The model under review builds one solid part; all positions refer to its coordinate system, in mm. A direction names the side the tool comes from. Give positions to 0.01 mm unless a question says otherwise; leave off trailing zeros. Loops run counter-clockwise (first coordinate to the right, second up) from the corner with the lowest first, then second, coordinate; pieces in that order, holes last. Notation, with made-up numbers: M 53,26 L 107,26 A16 ccw 107,47 Z; hole C 53,75.5 d8. An arc over 180 degrees is marked long. One line per item, written item: value. Start each with the question number.
Q1. Mouldability with a two-part tool opening along X and no side actions: class faces 3 (the face through (-30.2, 11.3, 0)), 4 (the face through (20.935, 16, -103)), 5 (the face through (-33.04, 14, -75)) as released by +X, released by -X, zero draft, split by the parting line, or undercut.
Q2. We need section C-C on x = -28. Write out the cut boundary in (y, z) (3 decimals).
Q3. For pin 1 (1 mm diameter, centred on x = -22.5, z = -66.5, fed in from +Y) (3 decimals); pin 2 (2 mm diameter, centred on y = 3.5, z = -43.5, fed in from +X); pin 3 (7.5 mm diameter, centred on y = 18.5, z = -52.5, fed in from +X), all flat-tipped, find the tip position at first contact; note any pin that passes through.
Q4. We need section B-B on z = -93.5. Write out the cut boundary in (x, y) (3 decimals), plus the area to 3 significant figures.
Q5. We need section D-D on z = -39.5. Write out the cut boundary in (x, y) (3 decimals), plus the area to 3 significant figures.
Q6. We need section A-A on y = 23. Write out the cut boundary in (x, z), plus the area to 3 significant figures.
Q7. For faces 1 (the face through (-5, 3.175, -92)), 2 (the face through (23, 28.575, -103)), list the 3-axis set-ups (+Z, -Z, +X, -X, +Y, -Y) from which the entire face can be reached by the end or side of a thin tool; tool diameter is ignored.
Q8. To check wall thickness, follow line 1 along X through (y, z) = (10, -85); line 2 along Y through (x, z) = (4, -50) (3 decimals); line 3 along X through (y, z) = (23.5, -7). State the ranges of each line that lie inside material, in increasing order. Write a range as from..to.
Autodesk Inventor part; units mm, degrees
ref_plane "YZ Plane" through (0, 0, 0) normal (1, 0, 0) x (0, 1, 0)
ref_plane "XZ Plane" through (0, 0, 0) normal (0, 1, 0) x (-1, 0, 0)
ref_plane "XY Plane" through (0, 0, 0) normal (0, 0, 1) x (1, 0, 0)
sketch "Sketch1" plane through (0, 0, 0) normal (0, 0, 1) x (1, 0, 0)
  line L0 (24.1101, 28.575) -> (24.1101, 0)
  line L1 (24.1101, 0) -> (-33.0399, 0)
  line L2 (-33.0399, 0) -> (-33.0399, 28.575)
  line L3 (-29.8649, 28.575) -> (-29.8649, 3.175)
  line L4 (-29.8649, 3.175) -> (20.9351, 3.175)
  line L5 (20.9351, 3.175) -> (20.9351, 28.575)
  line L6 (-33.0399, 28.575) -> (-29.8649, 28.575)
  line L7 (24.1101, 28.575) -> (20.9351, 28.575)
  point P0 (0, 0)
  dimension "d0" = 57.15
  dimension "d1" = 28.575
  dimension "d2" = 3.175
  dimension "d18" = 28.575
extrude "Extrusion1" add sketch "Sketch1" against normal blind 152.4
sketch "Sketch5" plane through (-33.0399, 0, 0) normal (0, -1, 0) x (1, 0, 0)
  line L0 (0, 0) -> (57.15, 0)
  line L1 (57.15, 0) -> (57.15, -152.4)
  line L2 (57.15, -152.4) -> (57.15, -59.69)
  line L3 (57.15, 0) -> (57.15, -152.4)
  line L4 (57.15, -59.69) -> (10.5151, 0)
  line L5 (10.5151, 0) -> (57.15, 0)
  line L6 (57.15, 0) -> (57.15, -59.69)
  point P0 (33.0399, 0)
  dimension "d14" = 92.71
  dimension "d15" = 38
extrude "Extrusion4" cut sketch "Sketch5" against normal through all
properties part number "Horizontal channel right" material "Aluminum 6061"
Solved:
1. face 3: zero draft
1. face 4: undercut
1. face 5: released by -X
2. outline: M 0,-152.4 L 3.175,-152.4 L 3.175,0 L 0,0 Z
3. pin 1: y = 3.175
3. pin 2: x = 12.2
3. pin 3: x = 21.42
4. outline: M -33.04,0 L 24.11,0 L 24.11,28.575 L 20.935,28.575 L 20.935,3.175 L -29.865,3.175 L -29.865,28.575 L -33.04,28.575 Z
4. area: 343 mm2
5. outline: M -33.04,0 L 8.336,0 L 8.336,3.175 L -29.865,3.175 L -29.865,28.575 L -33.04,28.575 Z
5. area: 212 mm2
6. outline: M -33.04,-152.4 L -29.86,-152.4 L -29.86,0 L -33.04,0 Z; M 20.94,-152.4 L 24.11,-152.4 L 24.11,-59.69 L 20.94,-55.63 Z
6. area: 785 mm2
7. face 1: +Z, -Z, +Y
7. face 2: +Z, -Z, +X, -X, +Y
8. line 1: -33.04..-29.86, 20.94..24.11
8. line 2: 0..3.175
8. line 3: -33.04..-29.86
